The drawing under review shows one solid part. Ordinate dimensions are in mm from its lowest x, y, z. Coordinates: 2 decimals unless noted, no trailing zeros. Write each loop counter-clockwise with the first axis right and the second up, starting at its lowest first coordinate (ties: lowest second). Pieces come first, ordered by that corner, then holes.
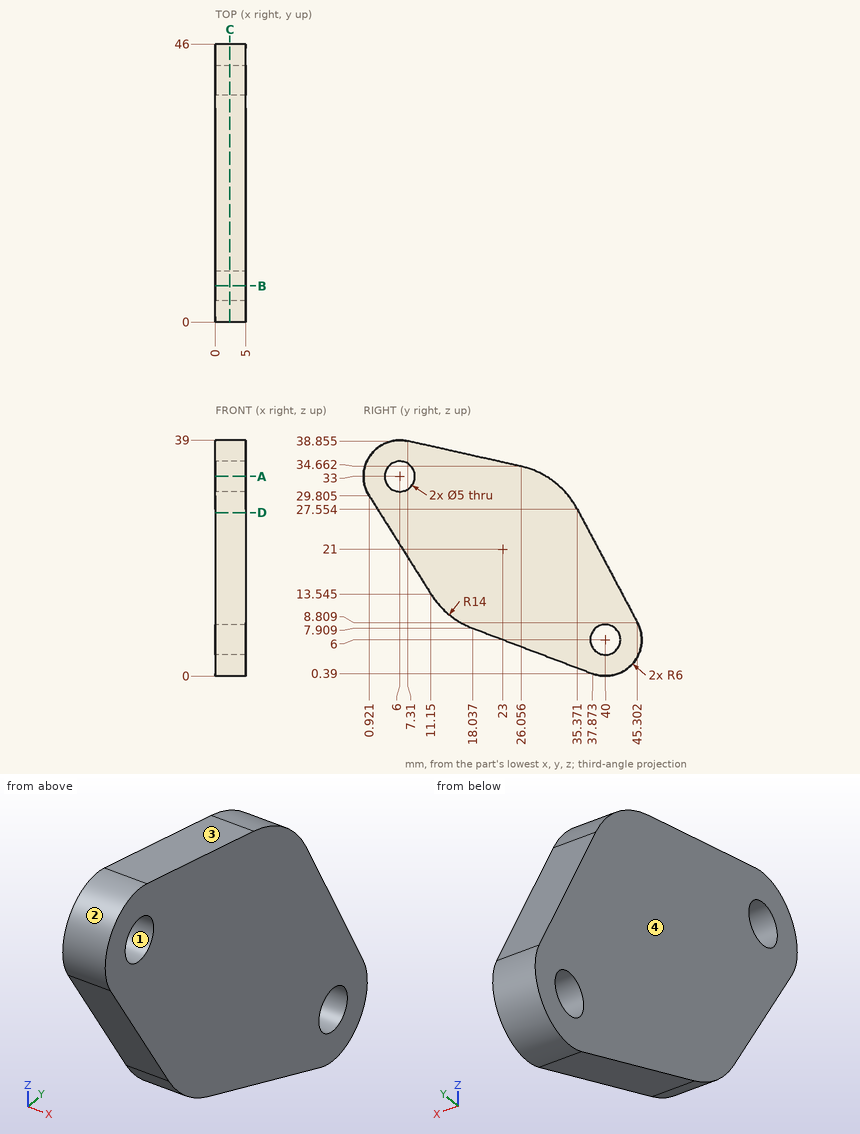
Q1. For probe 1 along Z at (x, y) = (3.2, 42) (1 decimal); probe 2 along Z at (x, y) = (1.7, 40) (1 decimal); probe 3 along Y at (x, z) = (0.5, 34) (1 decimal), list the stretches that pass through material, from the lowest coordinate up.
Ans:
probe 1: z = 0.3 to 4.5, 7.5 to 15
probe 2: z = 0 to 3.5, 8.5 to 18.8
probe 3: y = 0.1 to 3.7, 8.3 to 28.2
Q2. Draft analysis for pull direction Z (two halves, no side actions). For the marked faces 1, 2, 3 and 4, state which applies: +Z half, -Z half, draft (parallel to the pull), parting line (faces both ways), or undercut.
Ans:
face 1: undercut
face 2: parting line
face 3: +Z half
face 4: draft
Q3. Add section A-A (z = 33). State the section outline as (x, y) points, then the cut area to 3 significant figures.
Ans:
outline: (0, 0) - (5, 0) - (5, 3.5) - (0, 3.5) - close; (0, 8.5) - (5, 8.5) - (5, 30.21) - (0, 30.21) - close
area: 126 mm2
Q4. Add section D-D (z = 27). State the section outline as (x, y) points (1 decimal), then the cut area to 3 significant figures.
Ans:
outline: (0, 2.7) - (5, 2.7) - (5, 35.7) - (0, 35.7) - close
area: 165 mm2
Q5. Add section C-C (x = 2.4). Give the number of separate pieces and of enclosed holes in the cut face, then the cut area to 3 significant figures.
Ans:
separate pieces: 1
enclosed holes: 2
area: 1,000 mm2
Q6. Clearance check with flat-ended pins moving along their axes: pin 1 Ø3 at (x, z) = (4, 12.5) entering from +Y; pin 2 Ø3 at (x, z) = (0.5, 14) entering from -Y; pin 3 Ø2 at (x, z) = (1.5, 20.5) entering from +Y. State where each tip first meets the part, or that it passes through.
Ans:
pin 1: stops at y = 44.14
pin 2: stops at y = 9.92
pin 3: stops at y = 39.64
Q7. Add section B-B (y = 6). State the section outline as (x, z) points.
Ans:
outline: (0, 21.73) - (5, 21.73) - (5, 30.5) - (0, 30.5) - close; (0, 35.5) - (5, 35.5) - (5, 39) - (0, 39) - close
